The model under review builds one solid part; all positions refer to its coordinate system, in mm. Face numbers are marked on the shaded views. A direction names the side the tool comes from. Round coordinates to 2 decimals unless told otherwise and drop trailing zeros. Write each loop counter-clockwise with the first axis right and the second up, starting at its lowest first coordinate (ties: lowest second). Pieces come first, ordered by that corner, then holes. Notation, with made-up numbers: M 68.25,84.5 L 126.25,84.5 A28 ccw 126.25,115.5 Z; hole C 55.25,-22 d3. An arc over 180 degrees is marked long. One line per item, written item: value. Start each with the question number.
1) Take a section at B-B, the plane z = 47.5. Write out the cut boundary in (x, y).
2) Take a section at C-C, the plane z = 34. Write out the cut boundary in (x, y), and give its area (3 significant figures).
3) Take a section at D-D, the plane y = 15.5. Write out the cut boundary in (x, z), and give its area (3 significant figures).
4) Wall thickness on probe 1 along X at (y, z) = (36.5, 25); probe 2 along Y at (x, z) = (15, 45); probe 3 along Z at (x, y) = (21.5, 106.5): over which ranges is each line inside the solid? List them lowest first.
5) Take a section at A-A, the plane y = 70.5. Write out the cut boundary in (x, z).
6) Tool access review of the marked faces 4, 5 and 6: name each direction out of +Z, -Z, +X, -X, +Y, -Y from which nothing blocks a thin tool from reaching the whole face with its end or side.
7) Mouldability with a two-part tool opening along X and no side actions: class the marked faces 1, 2 and 3 as +X half, -X half, draft (parallel to the pull), parting line (faces both ways), or undercut.
8) For P1, Ø10, axis at x = 37, y = 42, coming from the -Z side; P2, Ø3, axis at x = 79, y = 84.5, coming from the -Z side, all flat-tipped, find the tip position at first contact; note any pin that passes through.
from build123d import *

# Parameters (mm, degrees)
ESQUISSE1_W                  = 86
ESQUISSE1_H                  = 94
BOSS_EXTRU_1_DEPTH           = 60
ESQUISSE2_W                  = 82
ESQUISSE2_H                  = 90
ENL_V_MAT_EXTRU_1_DEPTH      = 58
ESQUISSE3_W                  = 86
ESQUISSE3_H                  = 60
BOSS_EXTRU_2_DEPTH           = 18
ESQUISSE5_W                  = 82
ESQUISSE5_H                  = 56
ENL_V_MAT_EXTRU_2_DEPTH      = 18
ENL_V_MAT_EXTRU_3_DEPTH      = 154.427507312
ENL_V_MAT_EXTRU_3_DEPTH_BACK = 18
ESQUISSE7_W                  = 23
ESQUISSE7_H                  = 15.44
ESQUISSE8_W                  = 14.5
ESQUISSE8_H                  = 31
ENL_V_MAT_EXTRU_4_DEPTH      = 18
ESQUISSE11_W                 = 20.95
ESQUISSE11_H                 = 14.9
ENL_V_MAT_EXTRU_5_DEPTH      = 18
ESQUISSE12_R                 = 3.095
ENL_V_MAT_EXTRU_6_DEPTH      = 18
ESQUISSE15_R                 = 3
BOSS_EXTRU_3_DEPTH           = 18
ENL_V_MAT_EXTRU_7_DEPTH      = 1.3


with BuildPart() as part:
    # Esquisse1 → Boss.-Extru.1 (new body)
    with BuildSketch(Plane.XY):
        with Locations((43, 47)):
            Rectangle(ESQUISSE1_W, ESQUISSE1_H)
    extrude(amount=BOSS_EXTRU_1_DEPTH)

    # Esquisse2 → Enlèv. mat.-Extru.1 (cut)
    with BuildSketch(Plane.XY):
        with Locations((43, 47)):
            Rectangle(ESQUISSE2_W, ESQUISSE2_H)
    extrude(amount=ENL_V_MAT_EXTRU_1_DEPTH, mode=Mode.SUBTRACT)

    # Esquisse3 → Boss.-Extru.2 (add)
    with BuildSketch(Plane(origin=(0, 94, 0), x_dir=(1, 0, 0), z_dir=(0, 1, 0))):
        with Locations((43, -30)):
            Rectangle(ESQUISSE3_W, ESQUISSE3_H)
    extrude(amount=BOSS_EXTRU_2_DEPTH)

    # Esquisse5 → Enlèv. mat.-Extru.2 (cut)
    with BuildSketch(Plane(origin=(0, 92, 0), x_dir=(1, 0, 0), z_dir=(0, 1, 0))):
        with Locations((43, -30)):
            Rectangle(ESQUISSE5_W, ESQUISSE5_H)
    extrude(amount=ENL_V_MAT_EXTRU_2_DEPTH, mode=Mode.SUBTRACT)

    # Esquisse7 → Enlèv. mat.-Extru.3 (cut, two sides: drawn at the far end of the back side and taken through both)
    with BuildSketch(Plane(origin=(86, 0, 0), x_dir=(0, 0, -1), z_dir=(1, 0, 0)).offset(-ENL_V_MAT_EXTRU_3_DEPTH_BACK)):
        with Locations((-19.5, 70.77985545)):
            Rectangle(ESQUISSE7_W, ESQUISSE7_H)
    extrude(amount=ENL_V_MAT_EXTRU_3_DEPTH + ENL_V_MAT_EXTRU_3_DEPTH_BACK, mode=Mode.SUBTRACT)

    # Esquisse8 → Enlèv. mat.-Extru.4 (cut)
    with BuildSketch(Plane.ZY):
        with Locations((20.75, 63.5)):
            Rectangle(ESQUISSE8_W, ESQUISSE8_H)
    extrude(amount=-ENL_V_MAT_EXTRU_4_DEPTH, mode=Mode.SUBTRACT)

    # Esquisse11 → Enlèv. mat.-Extru.5 (cut)
    with BuildSketch(Plane(origin=(86, 0, 0), x_dir=(0, 0, -1), z_dir=(1, 0, 0))):
        with Locations((-30.534625058, 96.750653673)):
            Rectangle(ESQUISSE11_W, ESQUISSE11_H)
    extrude(amount=-ENL_V_MAT_EXTRU_5_DEPTH, mode=Mode.SUBTRACT)

    # Esquisse12 → Enlèv. mat.-Extru.6 (cut)
    with BuildSketch(Plane.XZ):
        with Locations(Location((36.461804468, 26.688728835, 0), (0, 0, 270))):
            Circle(ESQUISSE12_R)
    extrude(amount=-ENL_V_MAT_EXTRU_6_DEPTH, mode=Mode.SUBTRACT)

    # Esquisse15 → Boss.-Extru.3 (add)
    with BuildSketch(Plane(origin=(0, 0, 58), x_dir=(-1, 0, 0), z_dir=(0, 0, -1))):
        with Locations(Location((-77.525036721, 7.963761202, 0), (0, 0, 180))):
            Circle(ESQUISSE15_R)
        with Locations(Location((-8.474963279, 7.963761202, 0), (0, 0, 180))):
            Circle(ESQUISSE15_R)
        with Locations(Location((-77.525036721, 86.036238798, 0), (0, 0, 180))):
            Circle(ESQUISSE15_R)
        with Locations(Location((-8.474963279, 86.036238798, 0), (0, 0, 180))):
            Circle(ESQUISSE15_R)
    extrude(amount=BOSS_EXTRU_3_DEPTH)

    # Esquisse16 → Enlèv. mat.-Extru.7 (cut)
    # profile 1 of 6: a face of its own
    with BuildSketch(Plane.XY.offset(60)):
        Polygon((15.8952664, 56.22062268), (15.8952664, 66.22062268), (16.083567682, 66.22062268), (22.690138195, 58.350029732), (22.690138195, 66.22062268), (23.587574092, 66.22062268), (23.587574092, 56.22062268), (23.383247169, 56.22062268), (16.792702297, 64.073186783), (16.792702297, 56.22062268), align=None)
    # profile 2 of 6: a face of its own
    with BuildSketch(Plane.XY.offset(60)):
        Polygon((30.254240759, 66.22062268), (34.869625374, 56.22062268), (33.894064477, 56.22062268), (32.415699092, 59.425750886), (27.882445887, 59.425750886), (26.3640164, 56.22062268), (25.382445887, 56.22062268), (30.126035631, 66.22062268), align=None)
        Polygon((30.180122169, 64.269500886), (28.371227939, 60.451391911), (31.942942682, 60.451391911), align=None, mode=Mode.SUBTRACT)
    # profile 3 of 6: a face of its own
    with BuildSketch(Plane.XY.offset(60)):
        Polygon((35.510651015, 65.194981655), (35.510651015, 66.22062268), (40.767061272, 66.22062268), (40.767061272, 65.194981655), (38.587574092, 65.194981655), (38.587574092, 56.22062268), (37.690138195, 56.22062268), (37.690138195, 65.194981655), align=None)
    # profile 4 of 6: a face of its own
    with BuildSketch(Plane.XY.offset(60)):
        Polygon((42.30552281, 66.22062268), (43.202958708, 66.22062268), (43.202958708, 62.118058578), (48.331163836, 62.118058578), (48.331163836, 66.22062268), (49.228599733, 66.22062268), (49.228599733, 56.22062268), (48.331163836, 56.22062268), (48.331163836, 61.092417552), (43.202958708, 61.092417552), (43.202958708, 56.22062268), (42.30552281, 56.22062268), align=None)
    # profile 5 of 6: a face of its own
    with BuildSketch(Plane.XY.offset(60)):
        Polygon((55.8952664, 66.22062268), (60.510651015, 56.22062268), (59.535090118, 56.22062268), (58.056724733, 59.425750886), (53.523471528, 59.425750886), (52.005042041, 56.22062268), (51.023471528, 56.22062268), (55.767061272, 66.22062268), align=None)
        Polygon((55.82114781, 64.269500886), (54.01225358, 60.451391911), (57.583968323, 60.451391911), align=None, mode=Mode.SUBTRACT)
    # profile 6 of 6: a face of its own
    with BuildSketch(Plane.XY.offset(60)):
        Polygon((62.30552281, 56.22062268), (62.30552281, 66.22062268), (62.493824092, 66.22062268), (69.100394605, 58.350029732), (69.100394605, 66.22062268), (69.997830503, 66.22062268), (69.997830503, 56.22062268), (69.79350358, 56.22062268), (63.202958708, 64.073186783), (63.202958708, 56.22062268), align=None)
    extrude(amount=-ENL_V_MAT_EXTRU_7_DEPTH, mode=Mode.SUBTRACT)


solid = part.part
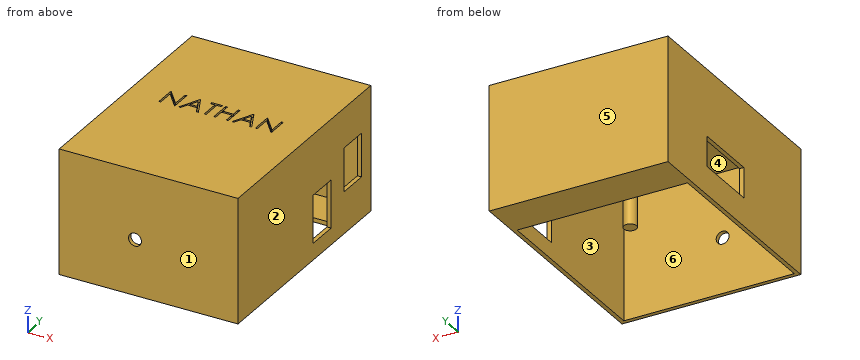
Checked values:
1. outline: M 0,0 L 86,0 L 86,112 L 0,112 Z; C 8.47,7.96 d6; C 8.47,86.04 d6; C 77.53,7.96 d6; C 77.53,86.04 d6; hole M 2,2 L 84,2 L 84,110 L 2,110 Z
2. outline: M 0,0 L 86,0 L 86,89.3 L 84,89.3 L 84,2 L 2,2 L 2,110 L 84,110 L 84,104.2 L 86,104.2 L 86,112 L 0,112 Z
2. area: 746 mm2
3. outline: M 0,0 L 2,0 L 2,58 L 84,58 L 84,0 L 86,0 L 86,60 L 0,60 Z
3. area: 404 mm2
4. probe 1: x = 0 to 2, 84 to 86
4. probe 2: y = 0 to 2, 110 to 112
4. probe 3: z = 0 to 2, 58 to 60
5. outline: M 0,0 L 2,0 L 2,13.5 L 0,13.5 Z; M 0,28 L 2,28 L 2,58 L 84,58 L 84,31 L 86,31 L 86,60 L 0,60 Z; M 84,0 L 86,0 L 86,8 L 84,8 Z
6. face 4: none
6. face 5: +Z, -Z, +X, -X, +Y
6. face 6: -Z
7. face 1: draft
7. face 2: +X half
7. face 3: undercut
8. P1: stops at z = 58
8. P2: stops at z = 40
